Input: part model. Units: mm. Frame: model coordinates. A direction names the side the tool comes from. Give positions to 0.01 mm unless a question says otherwise; leave off trailing zeros. Loops run counter-clockwise (first coordinate to the right, second up) from the corner with the lowest first, then second, coordinate; pieces in that order, holes last. Notation, with made-up numbers: M 88,67.25 L 93,67.25 A19 ccw 93,79.25 Z; hole C 9.5,-9.75 d7. An arc over 180 degrees is marked long. Use CSV: the item, a comma, the result in double quotes. Start each with the question number.
from build123d import *

# Parameters (mm, degrees)
SKETCH1_W                    = 190.5
SKETCH1_H                    = 101.6
BOSS_EXTRUDE1_DEPTH          = 3.175
SKETCH2_R                    = 14.2875
CUT_EXTRUDE1_DEPTH           = 3.175
EDGE_FLANGE1_STRIP_W         = 32.7
EDGE_FLANGE1_STRIP_H         = 3.175
EDGE_FLANGE1_STRIP_CUT_DEPTH = 190.5
EDGE_FLANGE1_DEPTH           = 190.5
SKETCH12_R                   = 9.525
SKETCH12_R_2                 = 2.54
CUT_EXTRUDE2_DEPTH           = 27.94
FILLET1_R                    = 38.1
SKETCH15_W                   = 3.175
SKETCH15_H                   = 25.4
BOSS_EXTRUDE2_DEPTH          = 0.000254
EDGE_FLANGE4_STRIP_W         = 32.7
EDGE_FLANGE4_STRIP_H         = 3.175
EDGE_FLANGE4_STRIP_CUT_DEPTH = 25.4
EDGE_FLANGE4_DEPTH           = 25.4
SKETCH26_R                   = 2.54
CUT_EXTRUDE3_DEPTH           = 142.028796748
SKETCH27_R                   = 2.54
CUT_EXTRUDE4_DEPTH           = 199.405991339
CUT_EXTRUDE5_START           = -34.29
CUT_EXTRUDE5_DEPTH           = 68.58
FILLET2_R                    = 2.54


# Read off the part's stored shape, not the designer's step: Cut-Extrude5
# Sheet-metal steps are written as plain solids
with BuildPart() as part:
    # Sketch1 → Boss-Extrude1 (new body)
    with BuildSketch(Plane(origin=(0, 0, 0), x_dir=(0, 0, -1), z_dir=(1, 0, 0))):
        Rectangle(SKETCH1_W, SKETCH1_H)
    extrude(amount=BOSS_EXTRUDE1_DEPTH)

    # Sketch2 → Cut-Extrude1 (cut)
    with BuildSketch(Plane(origin=(3.175, 0, 0), x_dir=(0, 0, -1), z_dir=(1, 0, 0))):
        with Locations((0, -25.4)):
            Circle(SKETCH2_R)
    extrude(amount=-CUT_EXTRUDE1_DEPTH, mode=Mode.SUBTRACT)

    # Edge-Flange1 strip (across the edge) → Edge-Flange1 strip cut (cut)
    with BuildSketch(Plane(origin=(0, 50.8, 95.25), x_dir=(0, -1, 0), z_dir=(0, 0, -1))):
        with Locations((-3.175, -1.5875)):
            Rectangle(EDGE_FLANGE1_STRIP_W, EDGE_FLANGE1_STRIP_H)
    extrude(amount=EDGE_FLANGE1_STRIP_CUT_DEPTH, mode=Mode.SUBTRACT)

    # Edge-Flange1 section (across the edge) → Edge-Flange1 (add)
    with BuildSketch(Plane(origin=(0, 50.8, 95.25), x_dir=(0, -1, 0), z_dir=(0, 0, -1))):
        with BuildLine():
            Line((0, 10), (0, 22.225))
            Line((0, 22.225), (3.175, 22.225))
            Line((3.175, 22.225), (3.175, 10))
            ThreePointArc((3.175, 10), (6.103932188, 2.928932188), (13.175, 0))
            Line((13.175, 0), (13.175, -3.175))
            ThreePointArc((13.175, -3.175), (3.858868158, 0.683868158), (0, 10))
        make_face()
    extrude(amount=EDGE_FLANGE1_DEPTH)

    # Sketch12 → Cut-Extrude2 (cut)
    with BuildSketch(Plane(origin=(3.175, 0, 0), x_dir=(0, 0, -1), z_dir=(1, 0, 0))):
        with Locations((-47.963329482, 12.225)):
            Circle(SKETCH12_R)
        with Locations((-28.616658964, 28.683017495)):
            Circle(SKETCH12_R_2)
        with Locations((-67.31, -4.233017495)):
            Circle(SKETCH12_R_2)
        with Locations((47.963329482, 12.225)):
            Circle(SKETCH12_R)
        with Locations((28.616658964, 28.683017495)):
            Circle(SKETCH12_R_2)
        with Locations((67.31, -4.233017495)):
            Circle(SKETCH12_R_2)
    extrude(amount=-CUT_EXTRUDE2_DEPTH, mode=Mode.SUBTRACT)

    # Fillet1
    fillet1_edges = [part.edges().sort_by_distance(p)[0] for p in [
        (1.5875, -50.8, 95.25),
        (1.5875, -50.8, -95.25),
    ]]
    fillet(fillet1_edges, radius=FILLET1_R)

    # Sketch15 → Boss-Extrude2 (add)
    with BuildSketch(Plane.XY.offset(95.25)):
        with Locations((1.5875, 6.35)):
            Rectangle(SKETCH15_W, SKETCH15_H)
    extrude(amount=BOSS_EXTRUDE2_DEPTH)

    # Edge-Flange4 strip (across the edge) → Edge-Flange4 strip cut (cut)
    with BuildSketch(Plane(origin=(0, -6.35, 95.250254), x_dir=(0, 0, -1), z_dir=(0, 1, 0))):
        with Locations((-3.175, -1.5875)):
            Rectangle(EDGE_FLANGE4_STRIP_W, EDGE_FLANGE4_STRIP_H)
    extrude(amount=EDGE_FLANGE4_STRIP_CUT_DEPTH, mode=Mode.SUBTRACT)

    # Edge-Flange4 section (across the edge) → Edge-Flange4 (add)
    with BuildSketch(Plane(origin=(0, -6.35, 95.250254), x_dir=(0, 0, -1), z_dir=(0, 1, 0))):
        with BuildLine():
            Line((0, 10), (0, 22.225))
            Line((0, 22.225), (3.175, 22.225))
            Line((3.175, 22.225), (3.175, 10))
            ThreePointArc((3.175, 10), (6.103932188, 2.928932188), (13.175, 0))
            Line((13.175, 0), (13.175, -3.175))
            ThreePointArc((13.175, -3.175), (3.858868158, 0.683868158), (0, 10))
        make_face()
    extrude(amount=EDGE_FLANGE4_DEPTH)

    # Sketch26 → Cut-Extrude3 (cut, through all)
    with BuildSketch(Plane(origin=(0, 50.8, 0), x_dir=(1, 0, 0), z_dir=(0, 1, 0))):
        with Locations(Location((-14.605, -82.55, 0), (0, 0, 180))):
            Circle(SKETCH26_R)
        with Locations(Location((-14.605, -64.205555556, 0), (0, 0, 180))):
            Circle(SKETCH26_R)
        with Locations(Location((-14.605, -45.861111111, 0), (0, 0, 180))):
            Circle(SKETCH26_R)
        with Locations(Location((-14.605, -27.516666667, 0), (0, 0, 180))):
            Circle(SKETCH26_R)
        with Locations(Location((-14.605, -9.172222222, 0), (0, 0, 180))):
            Circle(SKETCH26_R)
        with Locations(Location((-14.605, 9.172222222, 0), (0, 0, 180))):
            Circle(SKETCH26_R)
        with Locations(Location((-14.605, 27.516666667, 0), (0, 0, 180))):
            Circle(SKETCH26_R)
        with Locations(Location((-14.605, 45.861111111, 0), (0, 0, 180))):
            Circle(SKETCH26_R)
        with Locations(Location((-14.605, 64.205555556, 0), (0, 0, 180))):
            Circle(SKETCH26_R)
        with Locations(Location((-14.605, 82.55, 0), (0, 0, 180))):
            Circle(SKETCH26_R)
    extrude(amount=-CUT_EXTRUDE3_DEPTH, mode=Mode.SUBTRACT)

    # Sketch27 → Cut-Extrude4 (cut, through all)
    with BuildSketch(Plane.XY.offset(95.250254)):
        with Locations((-16.35, 12.7)):
            Circle(SKETCH27_R)
        with Locations((-16.35, 0)):
            Circle(SKETCH27_R)
    extrude(amount=-CUT_EXTRUDE4_DEPTH, mode=Mode.SUBTRACT)

    # Cut-Extrude5 outline → Cut-Extrude5 (cut)
    with BuildSketch(Plane.XY.offset(CUT_EXTRUDE5_START)):
        with BuildLine():
            ThreePointArc((-10, 47.625), (-9.762432951, 47.622177697), (-9.525, 47.61371238))
            Line((-9.525, 47.61371238), (-9.3741875, 50.78512856))
            ThreePointArc((-9.3741875, 50.78512856), (-9.687005413, 50.796281615), (-10, 50.8))
            Line((-10, 50.8), (-22.225, 50.8))
            Line((-22.225, 50.8), (-22.225, 47.625))
            Line((-22.225, 47.625), (-10, 47.625))
        make_face()
    extrude(amount=CUT_EXTRUDE5_DEPTH, mode=Mode.SUBTRACT)

    # Fillet2
    fillet2_edges = [part.edges().sort_by_distance(p)[0] for p in [
        (-22.225, 49.2125, 95.25),
        (-22.225, 49.2125, 34.29),
        (-9.44959375, 49.19942047, 34.29),
        (-9.44959375, 49.19942047, -34.29),
        (-22.225, 49.2125, -34.29),
        (-22.225, 49.2125, -95.25),
    ]]
    fillet(fillet2_edges, radius=FILLET2_R)


solid = part.part
Item 1: Mould query, pull axis X, two halves, no side actions, for faces 1 (the flat face through (0, -6, 1)), 2 (the flat face through (0, 40, 95.25)), 3 (the cylindrical face through (-14.05, 49.23, -85.03)), 4 (the flat face through (3.175, -6, 1)). Classes: +X half, -X half, draft (parallel to the pull), parting line (faces both ways), or undercut.
Item 2: Set-up query: faces 5 (the flat face through (-16, 6, 92.075)), 6 (the flat face through (-18, 47.625, -64)), 7 (the cylindrical face through (1.61, -39.34, -84.39)). Return all of +Z, -Z, +X, -X, +Y, -Y with unobstructed straight access to the full face (end or side cutting, diameter ignored); none if empty.
Item 3: First-contact query: pin 1 Ø4 at (x, y) = (-7.5, -4.5) entering from -Z; pin 2 Ø4 at (y, z) = (-29, 26.5) entering from -X; pin 3 Ø3.5 at (x, z) = (-14.5, 76) entering from -Y (3 decimals). Flat tips, straight axial feed; report the tip coordinate or a pass-through.
Item 4: Section B-B (x = -3). Output: boundary loops of the cut face in (y, z), then the cut area to 3 significant figures.
Item 5: Material intervals for line 1 (X direction, y = -40, z = -15.5) (3 decimals); line 2 (Y direction, x = -19.25, z = 74.5) (3 decimals); line 3 (X direction, y = 9.5, z = 83), sorted ascending.
Item 6: Section C-C (y = -25.4). Output: boundary loops of the cut face in (x, z) (1 decimal).
Item 7: Section D-D (z = -77). Output: boundary loops of the cut face in (x, y) (3 decimals).
Recorded:
1,face 1,"-X half"
1,face 2,"draft"
1,face 3,"undercut"
1,face 4,"+X half"
2,face 5,"-Z, -X, -Y"
2,face 6,"+Z, -Z, -X, -Y"
2,face 7,"-Z, +X, -X, -Y"
3,pin 1,"z = 91.01"
3,pin 2,"x = 0"
3,pin 3,"y = 47.625"
4,outline,"M -6.35,89.22 L 19.05,89.22 L 19.05,93.24 L -6.35,93.24 Z; M 44.77,-95.25 L 48.79,-95.25 L 48.79,95.25 L 44.77,95.25 Z"
4,area,"868 mm²"
5,line 1,"0 to 3.175"
5,line 2,"47.625 to 50.8"
5,line 3,"-0.04 to 3.14"
6,outline,"M 0,-93.1 L 3.2,-93.1 L 3.2,-14.3 L 0,-14.3 Z; M 0,14.3 L 3.2,14.3 L 3.2,93.1 L 0,93.1 Z"
7,outline,"M -22.225,47.625 L -10,47.625 A10 cw 0,37.625 L 0,-45.221 L 3.175,-45.221 L 3.175,37.625 A13.175 ccw -10,50.8 L -22.225,50.8 Z"
